Part model, mm, in its own coordinate system. A direction names the side the tool comes from. Coordinates: 2 decimals unless noted, no trailing zeros. Loops run counter-clockwise (first coordinate to the right, second up) from the corner with the lowest first, then second, coordinate; pieces in that order, holes last. Notation, with made-up numbers: (34, 30) - (83, 30) arc R32 cw to (83, 60) - close; hole circle Ø8 at (30.5, 31). An arc over 180 degrees is marked (long way). Answer as CSV lines item,"result".
from build123d import *

# Parameters (mm, degrees)
SKETCH009_R     = 2.65
SKETCH009_R_2   = 1.75
PAD003_DEPTH    = 6
SKETCH010_R     = 3.75
SKETCH010_R_2   = 2.65
PAD004_DEPTH    = 1
SKETCH011_R     = 3
POCKET006_DEPTH = 3


with BuildPart() as part:
    # Sketch009 (on Face6 of Binder) → Pad003 (new body)
    with BuildSketch(Plane.XY.offset(6)):
        with BuildLine():
            ThreePointArc((-13.4, 40.65), (-20.9, 33.15), (-13.4, 25.65))
            Line((-13.4, 25.65), (13.400012, 25.65))
            ThreePointArc((13.400012, 25.65), (20.9, 33.15), (13.400012, 40.65))
            Line((-13.4, 40.65), (13.400012, 40.65))
        make_face()
        with Locations((-13.4, 33.15)):
            Circle(SKETCH009_R, mode=Mode.SUBTRACT)
        with Locations((13.4, 33.15)):
            Circle(SKETCH009_R, mode=Mode.SUBTRACT)
        with Locations((0, 33.15)):
            Circle(SKETCH009_R_2, mode=Mode.SUBTRACT)
    extrude(amount=PAD003_DEPTH)

    # Sketch010 (on Face9 of Pad003) → Pad004 (join)
    with BuildSketch(Plane.XY.offset(12)):
        with Locations((-13.4, 33.15)):
            Circle(SKETCH010_R)
        with Locations((-13.4, 33.15)):
            Circle(SKETCH010_R_2, mode=Mode.SUBTRACT)
        with Locations((13.4, 33.15)):
            Circle(SKETCH010_R)
        with Locations((13.4, 33.15)):
            Circle(SKETCH010_R_2, mode=Mode.SUBTRACT)
    extrude(amount=PAD004_DEPTH)

    # Sketch011 (on Face5 of Pad004) → Pocket006 (cut)
    with BuildSketch(Plane.XY.offset(12)):
        with Locations((0, 33.15)):
            Circle(SKETCH011_R)
    extrude(amount=-POCKET006_DEPTH, mode=Mode.SUBTRACT)


solid = part.part
Q1. Two-plate mould, pull along Y, no slides. Class faces 3 (the face through (14.623, 30.799, 9.451)), 4 (the face through (14, 36, 13)), 5 (the face through (15.42, 36.31, 12.49)), 6 (the face through (0.81, 31.6, 7.48)): released by +Y, released by -Y, zero draft, split by the parting line, or undercut.
Results:
face 3,"undercut"
face 4,"zero draft"
face 5,"split by the parting line"
face 6,"undercut"
Q2. Saw through at A-A (z = 7.5). Give the cut face in (x, y), then the cut area to 3 significant figures.
Results:
outline,"(-13.4, 25.65) - (13.4, 25.65) arc R7.5 ccw to (13.4, 40.65) - (-13.4, 40.65) arc R7.5 ccw to start; hole circle Ø5.3 at (-13.4, 33.15); hole circle Ø3.5 at (0, 33.15); hole circle Ø5.3 at (13.4, 33.15)"
area,"525 mm^2"
Q3. Which spindle directions (+Z, -Z, +X, -X, +Y, -Y) get a long thin tool onto all of the face, cutting with end or side? Do faces 1 (the face through (-16, 32, 13)), 2 (the face through (1.61, 35.68, 10.52)). Say none if no direction does.
Results:
face 1,"+Z, +X, -X, +Y, -Y"
face 2,"+Z"
Q4. Saw through at D-D (z = 10). Give the cut face in (x, y), then the cut area to 3 significant figures.
Results:
outline,"(-13.4, 25.65) - (13.4, 25.65) arc R7.5 ccw to (13.4, 40.65) - (-13.4, 40.65) arc R7.5 ccw to start; hole circle Ø5.3 at (-13.4, 33.15); hole circle Ø6 at (0, 33.15); hole circle Ø5.3 at (13.4, 33.15)"
area,"506 mm^2"
Q5. Flat gauge pins, fed straight in: pin 1 (7 mm diameter, centred on x = 0, y = 33.15, fed in from +Z); pin 2 (5.5 mm diameter, centred on x = 0, y = 33.15, fed in from -Z); pin 3 (3 mm diameter, centred on x = 0.5, y = 33.5, fed in from +Z); pin 4 (1.5 mm diameter, centred on y = 37, z = 11.5, fed in from -X). Where does each tip first touch, or does it go through?
Results:
pin 1,"stops at z = 12"
pin 2,"stops at z = 6"
pin 3,"stops at z = 9"
pin 4,"stops at x = -20.23"
Q6. Saw through at C-C (y = 33.75). Give the cut face in (x, z), then the cut area to 3 significant figures.
Results:
outline,"(-20.88, 6) - (-15.98, 6) - (-15.98, 13) - (-17.1, 13) - (-17.1, 12) - (-20.88, 12) - close; (-10.82, 6) - (-1.64, 6) - (-1.64, 9) - (-2.94, 9) - (-2.94, 12) - (-9.7, 12) - (-9.7, 13) - (-10.82, 13) - close; (1.64, 6) - (10.82, 6) - (10.82, 13) - (9.7, 13) - (9.7, 12) - (2.94, 12) - (2.94, 9) - (1.64, 9) - close; (15.98, 6) - (20.88, 6) - (20.88, 12) - (17.1, 12) - (17.1, 13) - (15.98, 13) - close"
area,"166 mm^2"
Q7. Wall check: L1, parallel to X at y = 33, z = 10.5; L2, parallel to Y at x = 0, z = 8.25; L3, parallel to Y at x = -13.5, z = 12.5. Give the ranges that are in metal, low to high.
Results:
L1,"x = -20.9 to -16.05, -10.75 to -3, 3 to 10.75, 16.05 to 20.9"
L2,"y = 25.65 to 31.4, 34.9 to 40.65"
L3,"y = 29.4 to 30.5, 35.8 to 36.9"
Q8. Saw through at B-B (x = 0). Give the cut face in (y, z).
Results:
outline,"(25.65, 6) - (31.4, 6) - (31.4, 9) - (30.15, 9) - (30.15, 12) - (25.65, 12) - close; (34.9, 6) - (40.65, 6) - (40.65, 12) - (36.15, 12) - (36.15, 9) - (34.9, 9) - close"
